from build123d import *

# Parameters (mm, degrees)
BOX003_W        = 3
BOX003_H        = 3
BOX003_DEPTH    = 4.5
BOX002_W        = 3
BOX002_H        = 7
BOX002_DEPTH    = 6.5
CHAMFER005_SIZE = 1
CHAMFER006_SIZE = 1
CHAMFER007_SIZE = 0.4


with BuildPart() as cube003:
    # Box003 → Box003 (new body)
    with BuildSketch(Plane(origin=(-1.5, -1.5, 0), x_dir=(1, 0, 0), z_dir=(0, 0, 1))):
        with Locations((1.5, 1.5)):
            Rectangle(BOX003_W, BOX003_H)
    extrude(amount=BOX003_DEPTH)


with BuildPart() as obj1:
    # Box002 → Box002 (new body)
    with BuildSketch(Plane(origin=(-1.5, -3.5, 0), x_dir=(1, 0, 0), z_dir=(0, 0, 1))):
        with Locations((1.5, 3.5)):
            Rectangle(BOX002_W, BOX002_H)
    extrude(amount=BOX002_DEPTH)

    # Cut002: cut Cube003
    add(cube003.part, mode=Mode.SUBTRACT)

    # Chamfer005
    chamfer005_edges = [obj1.edges().sort_by_distance(p)[0] for p in [
        (0, 3.5, 6.5),
        (0, -3.5, 6.5),
    ]]
    chamfer(chamfer005_edges, length=CHAMFER005_SIZE)

    # Chamfer006
    chamfer006_edges = [obj1.edges().sort_by_distance(p)[0] for p in [
        (-1.5, 0, 4.5),
        (1.5, 0, 4.5),
    ]]
    chamfer(chamfer006_edges, length=CHAMFER006_SIZE)

    # Chamfer007
    chamfer007_edges = [obj1.edges().sort_by_distance(p)[0] for p in [
        (-1.5, 3.5, 2.75),
        (-1.5, 3, 6),
        (-1.5, 0, 6.5),
        (-1.5, -3, 6),
        (-1.5, -3.5, 2.75),
        (1.5, -3.5, 2.75),
        (1.5, -3, 6),
        (1.5, 0, 6.5),
        (1.5, 3.5, 2.75),
        (1.5, 3, 6),
    ]]
    chamfer(chamfer007_edges, length=CHAMFER007_SIZE)


with BuildPart() as obj1_1:
    # Chamfer007001 placement: moved
    add(obj1.part.moved(Location((-4, 10, 0))))


solid = obj1_1.part
Model file for the job. Use its own axes, mm. A direction names the side the tool comes from. Round coordinates to 2 decimals unless told otherwise and drop trailing zeros. Loops run counter-clockwise (first coordinate to the right, second up) from the corner with the lowest first, then second, coordinate; pieces in that order, holes last.
1. Band-saw the part on C-C, the plane y = 9.25. List the corners of the cut face in (x, z).
Check values:
outline: (-5.5, 5.5) - (-4.5, 4.5) - (-3.5, 4.5) - (-2.5, 5.5) - (-2.5, 6.1) - (-2.9, 6.5) - (-5.1, 6.5) - (-5.5, 6.1) - close
2. Tool access for faces 1 (the flat face through (-3, 10, 5)), 2 (the flat face through (-5, 10, 5)), 3 (the flat face through (-4, 6.5, 3)), 4 (the flat face through (-4, 10, 4.5)), 5 (the flat face through (-4, 7, 6)): list every direction of +Z, -Z, +X, -X, +Y, -Y with a clear straight run to the whole face (end or side of a thin tool).
Check values:
face 1: -Z, +X
face 2: -Z, -X
face 3: +Z, -Z, +X, -X, -Y
face 4: -Z, +X, -X
face 5: +Z, +X, -X, -Y
3. Band-saw the part on D-D, the plane x = -4.8. List the corners of the cut face in (y, z).
Check values:
outline: (6.5, 0) - (8.5, 0) - (8.5, 4.8) - (11.5, 4.8) - (11.5, 0) - (13.5, 0) - (13.5, 5.5) - (12.5, 6.5) - (7.5, 6.5) - (6.5, 5.5) - close
4. Band-saw the part on B-B, the plane x = -4.4. List the corners of the cut face in (y, z).
Check values:
outline: (6.5, 0) - (8.5, 0) - (8.5, 4.5) - (11.5, 4.5) - (11.5, 0) - (13.5, 0) - (13.5, 5.5) - (12.5, 6.5) - (7.5, 6.5) - (6.5, 5.5) - close
5. Drop flat-ended pins along their axis: P1, Ø1.1, axis at x = -4, y = 10.5, coming from the -Z side; P2, Ø1.5, axis at y = 9.5, z = 1.5, coming from the +X side. Give the stop position or say it passes through.
Check values:
P1: stops at z = 4.5
P2: passes through
6. Band-saw the part on A-A, the plane z = 1.5. List the corners of the cut face in (x, y).
Check values:
outline: (-5.5, 6.9) - (-5.1, 6.5) - (-2.9, 6.5) - (-2.5, 6.9) - (-2.5, 8.5) - (-5.5, 8.5) - close; (-5.5, 11.5) - (-2.5, 11.5) - (-2.5, 13.1) - (-2.9, 13.5) - (-5.1, 13.5) - (-5.5, 13.1) - close
7. Mould opens along Y. For faces 6 (the flat face through (-4, 13.5, 3)), 7 (the flat face through (-2.7, 7.15, 5.87)), 8 (the flat face through (-4, 8.5, 2)), 9 (the flat face through (-4, 13, 0)) say: +Y half, -Y half, draft (parallel to the pull), parting line (faces both ways), or undercut.
Check values:
face 6: +Y half
face 7: -Y half
face 8: undercut
face 9: draft
8. Wall check: probe 1 along Y at (x, z) = (-4.6, 2.25); probe 2 along Y at (x, z) = (-2.7, 2.5); probe 3 along Z at (x, y) = (-3.7, 8.75). Give the ranges that are in metal, low to high.
Check values:
probe 1: y = 6.5 to 8.5, 11.5 to 13.5
probe 2: y = 6.7 to 8.5, 11.5 to 13.3
probe 3: z = 4.5 to 6.5
